from build123d import *

# Parameters (mm, degrees)
ODGI_CIE_BAZOWE1_DEPTH          = 15
WYTNIJ_WYCI_GNI_CIE1_DEPTH      = 33.254612073
WYTNIJ_WYCI_GNI_CIE1_DEPTH_BACK = 1.6
SZKIC6_W                        = 2.3
SZKIC6_H                        = 1.6
SZKIC6_H_2                      = 13.2
WYTNIJ_WYCI_GNI_CIE2_REACH      = 34.255
SZKIC7_R                        = 2.6
SFAZOWANIE1_SIZE                = 3
ZAOKR_GLENIE1_R                 = 0.1
SFAZOWANIE2_SIZE                = 0.5


# Sheet-metal steps are written as plain solids
with BuildPart() as part:
    # Szkic1 → Odgięcie bazowe1 (new body)
    with BuildSketch(Plane.XY):
        with BuildLine():
            Line((0, 0), (0, 13.2))
            ThreePointArc((0, 13.2), (-0.234314575, 13.765685425), (-0.8, 14))
            Line((-0.8, 14), (-3.2, 14))
            ThreePointArc((-3.2, 14), (-4.33137085, 14.46862915), (-4.8, 15.6))
            Line((-4.8, 15.6), (-4.8, 28))
            Line((-4.8, 28), (-4, 28))
            Line((-4, 28), (-4, 15.6))
            ThreePointArc((-4, 15.6), (-3.765685425, 15.034314575), (-3.2, 14.8))
            Line((-3.2, 14.8), (-0.8, 14.8))
            ThreePointArc((-0.8, 14.8), (0.33137085, 14.33137085), (0.8, 13.2))
            Line((0.8, 13.2), (0.8, 0))
            Line((0.8, 0), (0, 0))
        make_face()
    extrude(amount=ODGI_CIE_BAZOWE1_DEPTH)

    # Szkic6 → Wytnij-wyciągnięcie1 (cut, two sides: drawn at the far end of the back side and taken through both)
    with BuildSketch(Plane(origin=(0.8, 0, 0), x_dir=(0, 0, -1), z_dir=(1, 0, 0)).offset(-WYTNIJ_WYCI_GNI_CIE1_DEPTH_BACK)):
        with Locations((-13.85, 14)):
            Rectangle(SZKIC6_W, SZKIC6_H)
        with Locations((-1.15, 14)):
            Rectangle(SZKIC6_W, SZKIC6_H)
        with Locations((-1.15, 6.6)):
            Rectangle(SZKIC6_W, SZKIC6_H_2)
        with Locations((-13.85, 6.6)):
            Rectangle(SZKIC6_W, SZKIC6_H_2)
    extrude(amount=WYTNIJ_WYCI_GNI_CIE1_DEPTH + WYTNIJ_WYCI_GNI_CIE1_DEPTH_BACK, mode=Mode.SUBTRACT)

    # Szkic7 → Wytnij-wyciągnięcie2 (cut, up to next)
    with BuildSketch(Plane.ZY.offset(4.8), mode=Mode.PRIVATE) as wytnij_wyci_gni_cie2_sk1:
        with Locations((7.5, 21.4)):
            Circle(SZKIC7_R)
    wytnij_wyci_gni_cie2_tool1 = extrude(wytnij_wyci_gni_cie2_sk1.sketch, amount=-WYTNIJ_WYCI_GNI_CIE2_REACH, mode=Mode.PRIVATE) & part.part
    add(wytnij_wyci_gni_cie2_tool1.solids().sort_by_distance((-4.8, 21.4, 7.5))[0], mode=Mode.SUBTRACT)

    # Sfazowanie1
    sfazowanie1_edges = [part.edges().sort_by_distance(p)[0] for p in [
        (-4.4, 28, 0),
        (-4.4, 28, 15),
    ]]
    chamfer(sfazowanie1_edges, length=SFAZOWANIE1_SIZE)

    # Zaokrąglenie1
    zaokr_glenie1_edges = [part.edges().sort_by_distance(p)[0] for p in [
        (-0.8, 14.4, 0),
        (-0.8, 14.4, 15),
    ]]
    fillet(zaokr_glenie1_edges, radius=ZAOKR_GLENIE1_R)

    # Sfazowanie2
    sfazowanie2_edges = [part.edges().sort_by_distance(p)[0] for p in [
        (0.4, 0, 2.3),
        (0.4, 0, 12.7),
    ]]
    chamfer(sfazowanie2_edges, length=SFAZOWANIE2_SIZE)


solid = part.part
Read the model definition and answer for the solid it produces. Units are mm, in the model's axes. A direction names the side the tool comes from. Coordinates: 2 decimals unless noted, no trailing zeros. Order: outer loops, then holes, each group sorted by start corner. A loop starts at its lowest first (then second) coordinate and runs counter-clockwise, first axis right, second up. Notation, with made-up numbers: (44, 3) - (87, 3) arc R22 ccw to (87, 23) - close; hole circle Ø9 at (45, 45). An arc over 180 degrees is marked (long way). Use one line per item in the form item = value.
(1) Which of the six approach directions +Z, -Z, +X, -X, +Y, -Y give full straight-line access (tool end or side, diameter ignored) to faces 4 (the face through (0, 7, 7)), 5 (the face through (-4.3, 18.7, 0)), 6 (the face through (-0.8, 14.4, 13.8)), 7 (the face through (0.3, 7.8, 2.3)), 8 (the face through (-4, 19, 9))?
Computed values:
face_4 = +Z, -Z, -X, -Y
face_5 = -Z, +X, -X, +Y, -Y
face_6 = +Z, +X, +Y, -Y
face_7 = -Z, +X, +Y, -Y
face_8 = +Z, -Z, +X, +Y
(2) Section A-A, the plane z = 8.5 is taken. Give the vertices of the cut face in (x, y).
Computed values:
outline = (-4.8, 15.6) arc R1.6 ccw to (-3.2, 14) - (-0.8, 14) arc R0.8 cw to (0, 13.2) - (0, 0) - (0.8, 0) - (0.8, 13.2) arc R1.6 ccw to (-0.8, 14.8) - (-3.2, 14.8) arc R0.8 cw to (-4, 15.6) - (-4, 19) - (-4.8, 19) - close; (-4.8, 23.8) - (-4, 23.8) - (-4, 28) - (-4.8, 28) - close
(3) Section B-B, the plane y = 21.4 is taken. Give the vertices of the cut face in (x, z), then the cut area to 3 significant figures.
Computed values:
outline = (-4.8, 0) - (-4, 0) - (-4, 4.9) - (-4.8, 4.9) - close; (-4.8, 10.1) - (-4, 10.1) - (-4, 15) - (-4.8, 15) - close
area = 7.84 mm²
(4) Given pin 1 Ø1.2 at (x, z) = (-2, 5) entering from -Y; pin 2 Ø0.7 at (x, z) = (-2.5, 10) entering from +Y; pin 3 Ø3 at (x, z) = (-2, 12) entering from +Y; pin 4 Ø1 at (x, y) = (-3, 24) entering from -Z, each flat-ended and moving along its own axis, determine where each tip first touches the part or whether it passes through.
Computed values:
pin_1 = 14
pin_2 = 14.8
pin_3 = 14.86
pin_4 = through
(5) For a pull along Y with two mould halves and no side action, classify faces 1 (the face through (-4.406, 19.093, 8.7)), 2 (the face through (-4.8, 24.5, 7.4)), 3 (the face through (-2, 14, 7)) as pulls with the +Y half, pulls with the -Y half, needs draft (parallel to the pull), parting line crosses it, or undercut.
Computed values:
face_1 = undercut
face_2 = needs draft
face_3 = pulls with the -Y half
(6) Straight lines are drawn through the part: L1, parallel to Y at x = -1.85, z = 10.25; L2, parallel to Y at x = -4.25, z = 7.5; L3, parallel to X at y = 7.75, z = 11.25. For each, find the intervals that lie inside material, in ascending order.
Computed values:
L1 = 14 to 14.8
L2 = 14.39 to 18.8, 24 to 28
L3 = 0 to 0.8
(7) Section C-C, the plane z = 13.5 is taken. Give the vertices of the cut face in (x, y), then the cut area to 3 significant figures.
Computed values:
outline = (-4.8, 15.6) arc R1.6 ccw to (-3.2, 14) - (-0.8, 14) - (-0.8, 14.8) - (-3.2, 14.8) arc R0.8 cw to (-4, 15.6) - (-4, 26.5) - (-4.8, 26.5) - close
area = 12.1 mm²
(8) Section D-D, the plane y = 12 is taken. Give the vertices of the cut face in (x, z), then the cut area to 3 significant figures.
Computed values:
outline = (0, 2.3) - (0.8, 2.3) - (0.8, 12.7) - (0, 12.7) - close
area = 8.32 mm²
